CAD build for the part. Positions are in the model's coordinates, mm. A direction names the side the tool comes from. Coordinates: 2 decimals unless noted, no trailing zeros. Loops run counter-clockwise (first coordinate to the right, second up) from the corner with the lowest first, then second, coordinate; pieces in that order, holes last. Notation, with made-up numbers: (11.25, 12) -> (23.25, 12) arc R20 ccw to (23.25, 29) -> close; hole circle Ø8 at (3, 60.5). An arc over 180 degrees is marked (long way). Return JSON: item names as keys, results as strings. Group by question number.
(1) Flat gauge pins, fed straight in: pin 1 Ø8 at (x, y) = (1, 2.5) entering from +Z; pin 2 Ø5 at (x, y) = (-5.5, 1.5) entering from +Z; pin 3 Ø4 at (x, z) = (-2.5, 5) entering from +Y. Where does each tip first touch, or does it go through?
(2) Mould opens along Y. For faces 5 (the face through (1.97, 0.62, 8.47)), 6 (the face through (-2, -6, -5)), 7 (the face through (-3, -1, -2)) say: pulls with the +Y half, pulls with the -Y half, needs draft (parallel to the pull), parting line crosses it, or undercut.
(3) Tool access for faces 1 (the face through (2.08, 0.65, 2.82)), 2 (the face through (-0.54, -2.44, 0.75)), 3 (the face through (1, -1, 10)), 4 (the face through (-5.75, 5.27, -3.23)): list every direction of +Z, -Z, +X, -X, +Y, -Y with a clear straight run to the whole face (end or side of a thin tool).
(4) Probe L1, parallel to Y at x = 0, z = -3.9; L2, parallel to Y at x = 0, z = 5.5; L3, parallel to X at y = -0.75, z = 7. List the from-to ranges inside material, lowest first.
(5) Saw through at A-A on z = 9.25. Write the cut outline in (x, y).
(6) Saw through at B-B on z = 6.5. Write the cut outline in (x, y), then the cut area to 3 significant figures.
```python
from build123d import *

# Parameters (mm, degrees)
SKETCH1_R                   = 2.5
SKETCH1_R_2                 = 1
BOSS_EXTRUDE1_DEPTH         = 5
CHAMFER2_SIZE               = 4
CHAMFER2_SIZE2              = 0.705307923
LPATTERN2_COUNT             = 2
LPATTERN2_PITCH             = 5
CHAMFER2_OF_LPATTERN2_SIZE2 = 0.705307923
CHAMFER2_OF_LPATTERN2_SIZE  = 4
FILLET1_R                   = 1
SKETCH2_R                   = 10
BOSS_EXTRUDE2_DEPTH         = 2
CUT_EXTRUDE2_START          = -15
SKETCH4_R                   = 1
CUT_EXTRUDE2_DEPTH          = 15
FILLET3_R                   = 2
SKETCH5_R                   = 7.8
SKETCH5_R_2                 = 6
BOSS_EXTRUDE3_DEPTH         = 5
FILLET4_R                   = 2
FILLET5_R                   = 0.5
FILLET6_R                   = 0.5


# Some blends are built 0.0001 mm under size
with BuildPart() as part:
    # Sketch1 → Boss-Extrude1 (new body)
    with BuildSketch(Plane.XY):
        Circle(SKETCH1_R)
        Circle(SKETCH1_R_2, mode=Mode.SUBTRACT)
    boss_extrude1 = extrude(amount=BOSS_EXTRUDE1_DEPTH)

    # Chamfer2
    chamfer2_edges = [part.edges().sort_by_distance(p)[0] for p in [
        (-2.5, 0, 5),
    ]]
    chamfer2_side = [part.faces().sort_by_distance(p)[0] for p in [
        (-2.5, 0, 2.5),
    ]]
    chamfer(chamfer2_edges, length=CHAMFER2_SIZE, length2=CHAMFER2_SIZE2, reference=chamfer2_side[0])


with BuildPart() as lpattern2_1:
    # LPattern2: Boss-Extrude1 ×2
    with Locations(*[(0, 0, i * LPATTERN2_PITCH) for i in range(1, LPATTERN2_COUNT)]):
        add(boss_extrude1)

    # Chamfer2 of LPattern2
    chamfer2_of_lpattern2_edges = [lpattern2_1.edges().sort_by_distance(p)[0] for p in [
        (-2.5, 0, 10),
    ]]
    chamfer(chamfer2_of_lpattern2_edges, length=CHAMFER2_OF_LPATTERN2_SIZE, length2=CHAMFER2_OF_LPATTERN2_SIZE2)


with BuildPart() as part_1:
    add(part.part)

    # LPattern2 united with what the copies to: union LPattern2_1
    add(lpattern2_1.part)

    # Fillet1
    # the kernel refuses this fillet: 1 mm, written as the material it adds along each edge
    with BuildSketch(Plane(origin=(0, 0, 5), x_dir=(1, 0, 0), z_dir=(0, -1, 0))) as fillet1_piece_1:
        with BuildLine():
            CenterArc((2.96611905, -0.884722008), FILLET1_R, 117.782669079, 72.217330921)
            Line((1.981311297, -1.058370186), (1.961615141, -1.061843149))
            Line((1.961615141, -1.061843149), (1.774995922, -0.003472964))
            Line((1.774995922, -0.003472964), (1.794692077, 0.02))
            ThreePointArc((1.794692077, 0.02), (2.147346039, 0.02), (2.490677619, 0.01769444))
            Line((2.490677619, 0.01769444), (2.5, 0))
        make_face()
    revolve(axis=Axis((0, 0, 5), (0, 0, 1)))

    # Sketch2 → Boss-Extrude2 (add)
    with BuildSketch(Plane.XY):
        Circle(SKETCH2_R)
    extrude(amount=-BOSS_EXTRUDE2_DEPTH)

    # Sketch4 → Cut-Extrude2 (cut)
    with BuildSketch(Plane.XY.offset(CUT_EXTRUDE2_START)):
        Circle(SKETCH4_R)
    extrude(amount=CUT_EXTRUDE2_DEPTH, mode=Mode.SUBTRACT)

    # Fillet3
    fillet3_edges = [part_1.edges().sort_by_distance(p)[0] for p in [
        (-1, 0, -2),
    ]]
    fillet(fillet3_edges, radius=FILLET3_R)

    # Sketch5 → Boss-Extrude3 (add)
    with BuildSketch(Plane.XY):
        Circle(SKETCH5_R)
        Circle(SKETCH5_R_2, mode=Mode.SUBTRACT)
    extrude(amount=-BOSS_EXTRUDE3_DEPTH)

    # Fillet4
    fillet4_edges = [part_1.edges().sort_by_distance(p)[0] for p in [
        (-10, 0, 0),
    ]]
    fillet(fillet4_edges, radius=FILLET4_R - 0.0001)  # a hair under: the kernel refuses the full size

    # Fillet5
    fillet5_edges = [part_1.edges().sort_by_distance(p)[0] for p in [
        (-2.5, 0, 0),
    ]]
    fillet(fillet5_edges, radius=FILLET5_R)

    # Fillet6
    fillet6_edges = [part_1.edges().sort_by_distance(p)[0] for p in [
        (-7.8, 0, -5),
    ]]
    fillet(fillet6_edges, radius=FILLET6_R)


solid = part_1.part
```
Geometry results:
{
 "1": {"pin 1": "z = 10", "pin 2": "z = 0", "pin 3": "y = 2.45"},
 "2": {"face 5": "parting line crosses it", "face 6": "needs draft", "face 7": "undercut"},
 "3": {"face 1": "none", "face 2": "+Z", "face 3": "+Z, +X, -X, +Y, -Y", "face 4": "-Z"},
 "4": {"L1": "-7.8 to -6, 6 to 7.8", "L2": "-2.5 to -1, 1 to 2.5", "L3": "-2.2 to -0.66, 0.66 to 2.2"},
 "5": {"outline": "circle Ø3.85 at (0, 0); hole circle Ø2 at (0, 0)"},
 "6": {"outline": "circle Ø4.82 at (0, 0); hole circle Ø2 at (0, 0)", "area": "15.1 mm²"}
}
